Part print with two shaded views. Sizes in mm from the minimum x, y, z corner. Round coordinates to 2 decimals unless told otherwise and drop trailing zeros. Order: outer loops, then holes, each group sorted by start corner. A loop starts at its lowest first (then second) coordinate and runs counter-clockwise, first axis right, second up. Notation, with made-up numbers: (-21.75, 11.5) -> (-6.75, 11.5) arc R11 cw to (-6.75, 23.5) -> close; hole circle Ø5 at (2, 0.5). An arc over 180 degrees is marked (long way). Use a Markdown table: item, result. Add a question column.
Item 1: Probe L1, parallel to X at y = 2, z = 2.15 (1 decimal); L2, parallel to X at y = 6.25, z = 0.8 (1 decimal); L3, parallel to Y at x = 27.5, z = 1.3. List the from-to ranges inside material, lowest first.
Item 2: Slice it at B-B, the plane y = 3.75. State how many separate pieces and enclosed holes the cut face has.
Item 3: Slice it at A-A, the plane z = 1.8. Give the cut face in (x, y) (1 decimal), plus the area to 3 significant figures.
Item 4: Two-plate mould, pull along Y, no slides. Class the marked faces 1, 2, 3 and 4: released by +Y, released by -Y, zero draft, split by the parting line, or undercut.
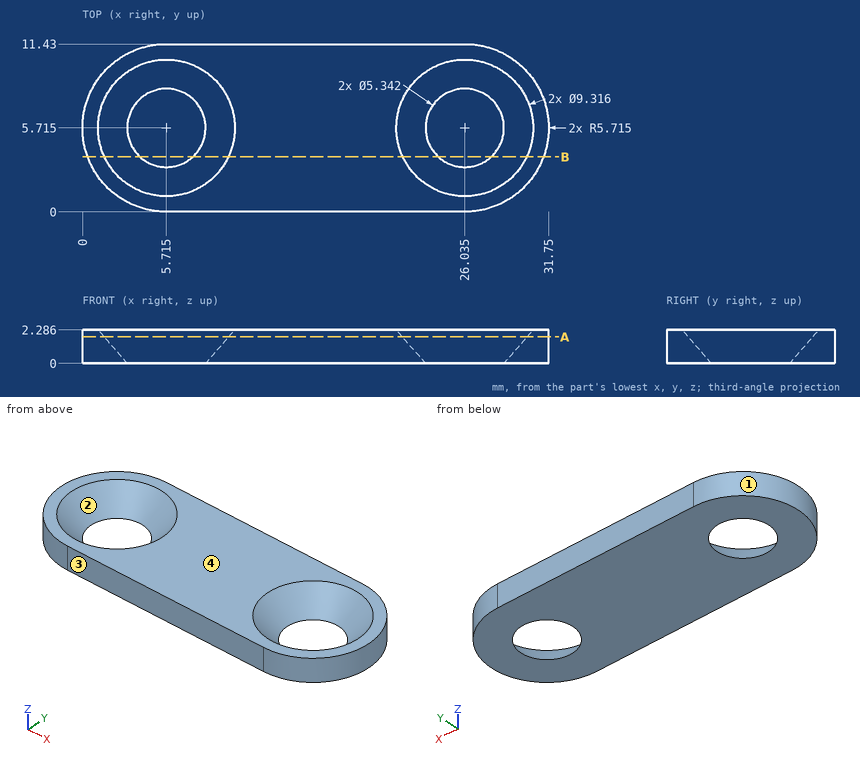
Check sheet entries:
| question | item | result |
|---|---|---|
| 1 | L1 | 1.4 to 3.1, 8.3 to 23.4, 28.6 to 30.4 |
| 1 | L2 | 0 to 2.4, 9 to 22.7, 29.4 to 31.7 |
| 1 | L3 | 0.19 to 2.21, 9.22 to 11.24 |
| 2 | separate pieces | 3 |
| 2 | enclosed holes | 0 |
| 3 | outline | (5.7, 0) -> (26, 0) arc R5.7 ccw to (26, 11.4) -> (5.7, 11.4) arc R5.7 ccw to start; hole circle Ø8.5 at (5.7, 5.7); hole circle Ø8.5 at (26, 5.7) |
| 3 | area | 222 mm2 |
| 4 | face 1 | split by the parting line |
| 4 | face 2 | undercut |
| 4 | face 3 | released by -Y |
| 4 | face 4 | zero draft |
